Verification items for the finished model (mm, model axes). A direction names the side the tool comes from. Coordinates: 2 decimals unless noted, no trailing zeros. Order: outer loops, then holes, each group sorted by start corner. A loop starts at its lowest first (then second) coordinate and runs counter-clockwise, first axis right, second up. Notation, with made-up numbers: (71.5, -3.5) -> (80.5, -3.5) arc R15 ccw to (80.5, 0.5) -> close; hole circle Ø1 at (61.5, 18). An arc over 180 degrees is marked (long way). Answer as CSV lines item,"result".
Autodesk Inventor part; units mm, degrees
ref_plane "YZ Plane" through (0, 0, 0) normal (1, 0, 0) x (0, 1, 0)
ref_plane "XZ Plane" through (0, 0, 0) normal (0, 1, 0) x (-1, 0, 0)
ref_plane "XY Plane" through (0, 0, 0) normal (0, 0, 1) x (1, 0, 0)
sketch "Sketch1" plane through (0, 0, 0) normal (0, 1, 0) x (-1, 0, 0)
  circle A0 centre (0, 0) radius 8 construction
  circle A1 centre (0, 0) radius 3
  line L0 (45, 15) -> (-45, 15)
  line L1 (-45, 15) -> (-45, -15)
  line L2 (-45, -15) -> (45, -15)
  line L3 (45, -15) -> (45, 15)
  line L4 (0, -21) -> (0, 21)
  point P0 (0, 15)
  dimension "d0" = 16
  dimension "d3" = 6
  dimension "d4" = 90
  dimension "d5" = 30
  dimension "d6" = 15
extrude "Extrusion1" add sketch "Sketch1" along normal blind 2.5 contours A1 L4 L0 L3 L2 | A1 L4 L2 L1 L0
sketch "Sketch2" plane through (0, 2.5, 0) normal (0, 1, 0) x (1, 0, 0)
  line L0 (-45, 15) -> (-45, -15)
  line L1 (-45, -15) -> (45, -15)
  line L2 (45, -15) -> (45, 15)
  line L3 (45, 15) -> (-45, 15)
  circle A0 centre (0, 0) radius 3
extrude "Extrusion2" add sketch "Sketch2" along normal blind 1
sketch "Sketch7" plane through (0, 0, 0) normal (0, -1, 0) x (1, 0, 0)
  circle A0 centre (-40, 10) radius 4
  line L0 (-45, 15) -> (45, 15)
  line L1 (-45, -15) -> (-45, 15)
  circle A1 centre (40, 10) radius 4
  circle A2 centre (-40, -10) radius 4
  circle A3 centre (40, -10) radius 4
  point P0 (0, 0)
  dimension "d34" = 8
  dimension "d35" = 5
  dimension "d36" = 5
  dimension "d39" = 80
  dimension "d42" = 20
extrude "Extrusion4" cut sketch "Sketch7" against normal blind 1
sketch "Sketch9" plane through (0, 3.5, 0) normal (0, 1, 0) x (1, 0, 0)
  circle A0 centre (-40, -10) radius 4 construction
  point P0 (0, 0)
hole "Hole2" at (-40, 3.5, 10) direction (0, -1, 0) diameter 3.4 end through all
pattern_linear "Rectangular Pattern1" count 2 spacing 20 along (0, 0, -1) count 2 spacing 80 along (1, 0, 0) of "Hole2"
chamfer "Chamfer2" distance 0.25 angle 45 1 edges at (-3, 3.5, 0)
sketch "Sketch11" plane through (0, 3.5, 0) normal (0, 1, 0) x (1, 0, 0)
  line L0 (-25, 0) -> (25, 0) construction
  point P0 (0, 0)
  point P1 (0, 0)
  dimension "d73" = 50
hole "Hole3" at (-25, 3.5, 0) at (25, 3.5, 0) direction (0, -1, 0) diameter 3.4 end through all
fillet "Fillet1" radius 2 4 edges at (-45, 1.75, 15) (45, 1.75, 15) (45, 1.75, -15) (-45, 1.75, -15)
properties part number "motor mount plate  for print"
Item 1: Section check A-A, the plane z = 0. Record the boundary of the cut face in (x, y).
Answer list:
outline,"(-45, 0) -> (-26.7, 0) -> (-26.7, 3.5) -> (-45, 3.5) -> close; (-23.3, 0) -> (-3, 0) -> (-3, 3.25) -> (-3.25, 3.5) -> (-23.3, 3.5) -> close; (3, 0) -> (23.3, 0) -> (23.3, 3.5) -> (3.25, 3.5) -> (3, 3.25) -> close; (26.7, 0) -> (45, 0) -> (45, 3.5) -> (26.7, 3.5) -> close"
Item 2: Section check D-D, the plane x = -40. Record the boundary of the cut face in (y, z), plus the area to 3 significant figures.
Answer list:
outline,"(0, -15) -> (3.5, -15) -> (3.5, -11.7) -> (1, -11.7) -> (1, -14) -> (0, -14) -> close; (0, -6) -> (1, -6) -> (1, -8.3) -> (3.5, -8.3) -> (3.5, 8.3) -> (1, 8.3) -> (1, 6) -> (0, 6) -> close; (0, 14) -> (1, 14) -> (1, 11.7) -> (3.5, 11.7) -> (3.5, 15) -> (0, 15) -> close"
area,"72.0 mm2"
Item 3: Thickness scan on line 1 (X direction, y = 0.6, z = 0.25); line 2 (Z direction, x = -25, y = 1.95); line 3 (X direction, y = 1.6, z = -10). Record the ranges inside material, lowest first.
Answer list:
line 1,"-45 to -26.68, -23.32 to -2.99, 2.99 to 23.32, 26.68 to 45"
line 2,"-15 to -1.7, 1.7 to 15"
line 3,"-45 to -41.7, -38.3 to 38.3, 41.7 to 45"
Item 4: Release check for a two-part mould opening along Z. For faces 1 (the cylindrical face through (41.66, 2.23, 9.63)), 2 (the cylindrical face through (-44.43, 1.77, 14.4)), 3 (the flat face through (1, 2, -15)), 4 (the flat face through (-45, 2, 0)) record: +Z half, -Z half, draft (parallel to the pull), parting line (faces both ways), or undercut.
Answer list:
face 1,"undercut"
face 2,"+Z half"
face 3,"-Z half"
face 4,"draft"
Item 5: Tool access check on faces 5 (the cylindrical face through (44.43, 1.73, 14.4)), 6 (the flat face through (-38, 1, -10)). Record the directions out of +Z, -Z, +X, -X, +Y, -Y that give a thin tool (end or side, any length) a straight path to the whole face; none if there is none.
Answer list:
face 5,"+Z, +X, +Y, -Y"
face 6,"-Y"
Item 6: Depth check by flat-ended pin: pin 1 Ø5.5 at (x, z) = (40, -10) entering from +Y; pin 2 Ø4 at (x, z) = (40.5, 11) entering from -Y. Enter the tip coordinate at first touch or a pass-through.
Answer list:
pin 1,"y = 3.5"
pin 2,"y = 1"
Item 7: Section check C-C, the plane x = 0. Record the boundary of the cut face in (y, z), plus the area to 3 significant figures.
Answer list:
outline,"(0, -15) -> (3.5, -15) -> (3.5, -3.25) -> (3.25, -3) -> (0, -3) -> close; (0, 3) -> (3.25, 3) -> (3.5, 3.25) -> (3.5, 15) -> (0, 15) -> close"
area,"83.9 mm2"
Item 8: Section check B-B, the plane y = 1.6. Record the boundary of the cut face in (x, z).
Answer list:
outline,"(-45, -13) arc R2 ccw to (-43, -15) -> (43, -15) arc R2 ccw to (45, -13) -> (45, 13) arc R2 ccw to (43, 15) -> (-43, 15) arc R2 ccw to (-45, 13) -> close; hole circle Ø3.4 at (-40, -10); hole circle Ø3.4 at (-40, 10); hole circle Ø3.4 at (-25, 0); hole circle Ø6 at (0, 0); hole circle Ø3.4 at (25, 0); hole circle Ø3.4 at (40, -10); hole circle Ø3.4 at (40, 10)"
